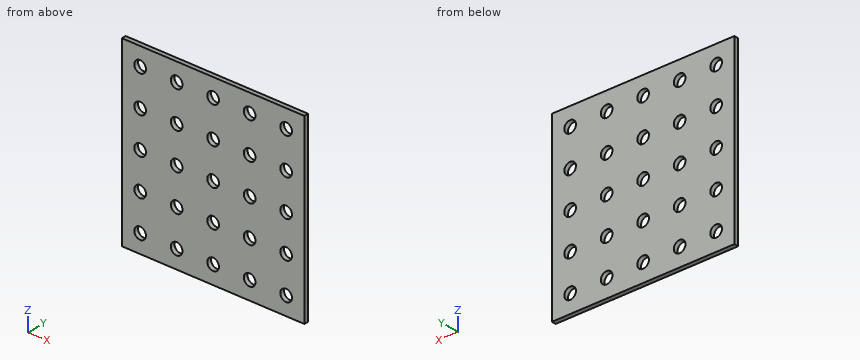
```python
from build123d import *

# Parameters (mm, degrees)
SKETCH_1_W          = 250
SKETCH_1_H          = 250
EXTRUDE_1_DEPTH     = 6
SKETCH_2_R          = 8
CUT_EXTRUDE_1_DEPTH = 6


with BuildPart() as part:
    # Эскиз1 → Бобышка-Вытянуть1 (new body)
    with BuildSketch(Plane(origin=(0, 0, 0), x_dir=(1, 0, 0), z_dir=(0, 1, 0))):
        Rectangle(SKETCH_1_W, SKETCH_1_H)
    extrude(amount=EXTRUDE_1_DEPTH)

    # Эскиз2 → Вырез-Вытянуть1 (cut)
    with BuildSketch(Plane(origin=(0, 6, 0), x_dir=(1, 0, 0), z_dir=(0, 1, 0))):
        with Locations((-100, -100)):
            Circle(SKETCH_2_R)
        with Locations((-50, -100)):
            Circle(SKETCH_2_R)
        with Locations((0, -100)):
            Circle(SKETCH_2_R)
        with Locations((50, -100)):
            Circle(SKETCH_2_R)
        with Locations((100, -100)):
            Circle(SKETCH_2_R)
        with Locations((-50, -50)):
            Circle(SKETCH_2_R)
        with Locations((0, -50)):
            Circle(SKETCH_2_R)
        with Locations((50, -50)):
            Circle(SKETCH_2_R)
        with Locations((100, -50)):
            Circle(SKETCH_2_R)
        with Locations((-50, 0)):
            Circle(SKETCH_2_R)
        Circle(SKETCH_2_R)
        with Locations((50, 0)):
            Circle(SKETCH_2_R)
        with Locations((100, 0)):
            Circle(SKETCH_2_R)
        with Locations((-50, 50)):
            Circle(SKETCH_2_R)
        with Locations((0, 50)):
            Circle(SKETCH_2_R)
        with Locations((50, 50)):
            Circle(SKETCH_2_R)
        with Locations((100, 50)):
            Circle(SKETCH_2_R)
        with Locations((-50, 100)):
            Circle(SKETCH_2_R)
        with Locations((0, 100)):
            Circle(SKETCH_2_R)
        with Locations((50, 100)):
            Circle(SKETCH_2_R)
        with Locations((100, 100)):
            Circle(SKETCH_2_R)
        with Locations((-100, -50)):
            Circle(SKETCH_2_R)
        with Locations((-100, 0)):
            Circle(SKETCH_2_R)
        with Locations((-100, 50)):
            Circle(SKETCH_2_R)
        with Locations((-100, 100)):
            Circle(SKETCH_2_R)
    extrude(amount=-CUT_EXTRUDE_1_DEPTH, mode=Mode.SUBTRACT)


solid = part.part
```
Can you work these out from the model? Positions are in its coordinate system, mm. Round coordinates to 2 decimals unless told otherwise and drop trailing zeros. Loops run counter-clockwise (first coordinate to the right, second up) from the corner with the lowest first, then second, coordinate; pieces in that order, holes last. Notation, with made-up numbers: (60.5, -26.75) -> (87.5, -26.75) arc R25 ccw to (87.5, 10.25) -> close; hole circle Ø7 at (5.5, 20). An arc over 180 degrees is marked (long way). One line per item, written item: value. Start each with the question number.
1. If I drill on probe 1 along X at (y, z) = (2.05, 100); probe 2 along X at (y, z) = (0.5, 44), over which ranges is the centre line in solid material (lowest first)?
2. If we section it at C-C, the plane y = 1.55: Give the number of separate pieces and of enclosed holes in the cut face, then the cut area to 3 significant figures.
3. If we section it at B-B, the plane z = 50: Write out the boundary of the cut face in (x, y).
4. For pin 1 (14.5 mm diameter, centred on x = 100, z = -50, fed in from +Y), with a flat end and sliding along its axis, tell me the tip position at first contact or that it passes through.
5. If we section it at A-A, the plane x = 0: Write out the boundary of the cut face in (y, z).
Calculated:
1. probe 1: x = -125 to -108, -92 to -58, -42 to -8, 8 to 42, 58 to 92, 108 to 125
1. probe 2: x = -125 to -105.29, -94.71 to -55.29, -44.71 to -5.29, 5.29 to 44.71, 55.29 to 94.71, 105.29 to 125
2. separate pieces: 1
2. enclosed holes: 25
2. area: 57,500 mm²
3. outline: (-125, 0) -> (-108, 0) -> (-108, 6) -> (-125, 6) -> close; (-92, 0) -> (-58, 0) -> (-58, 6) -> (-92, 6) -> close; (-42, 0) -> (-8, 0) -> (-8, 6) -> (-42, 6) -> close; (8, 0) -> (42, 0) -> (42, 6) -> (8, 6) -> close; (58, 0) -> (92, 0) -> (92, 6) -> (58, 6) -> close; (108, 0) -> (125, 0) -> (125, 6) -> (108, 6) -> close
4. pin 1: passes through
5. outline: (0, -125) -> (6, -125) -> (6, -108) -> (0, -108) -> close; (0, -92) -> (6, -92) -> (6, -58) -> (0, -58) -> close; (0, -42) -> (6, -42) -> (6, -8) -> (0, -8) -> close; (0, 8) -> (6, 8) -> (6, 42) -> (0, 42) -> close; (0, 58) -> (6, 58) -> (6, 92) -> (0, 92) -> close; (0, 108) -> (6, 108) -> (6, 125) -> (0, 125) -> close
